Autodesk Inventor part; units mm, degrees
ref_plane "YZ Plane" through (0, 0, 0) normal (1, 0, 0) x (0, 1, 0)
ref_plane "XZ Plane" through (0, 0, 0) normal (0, 1, 0) x (-1, 0, 0)
ref_plane "XY Plane" through (0, 0, 0) normal (0, 0, 1) x (1, 0, 0)
sketch "Sketch1" plane through (0, 0, 0) normal (0, 1, 0) x (-1, 0, 0)
  line L0 (0, 0) -> (127, 0)
  line L1 (127, 0) -> (127, -25.4)
  line L2 (127, -25.4) -> (0, -25.4)
  line L3 (0, -25.4) -> (0, 0)
  dimension "d0" = 127
  dimension "d1" = 25.4
extrude "Extrusion1" add sketch "Sketch1" along normal blind 7.62
sketch "Sketch2" plane through (0, 7.62, 0) normal (0, 1, 0) x (1, 0, 0)
  circle A0 centre (-17.78, 12.7) radius 6.2865
  circle A1 centre (-35.56, 12.7) radius 6.35
  circle A2 centre (-53.34, 12.7) radius 6.4135
  circle A3 centre (-71.12, 12.7) radius 6.477
  circle A4 centre (-88.9, 12.7) radius 6.5405
  circle A5 centre (-106.68, 12.7) radius 6.604
  line L0 (0, 0) -> (0, 25.4)
  dimension "d4" = 12.573
  dimension "d5" = 12.7
  dimension "d6" = 12.827
  dimension "d7" = 12.954
  dimension "d8" = 13.081
  dimension "d9" = 13.208
  dimension "d10" = 17.78
  dimension "d11" = 17.78
  dimension "d12" = 17.78
  dimension "d13" = 17.78
  dimension "d14" = 17.78
  dimension "d15" = 17.78
extrude "Extrusion2" cut sketch "Sketch2" against normal through all
fillet "Fillet1" radius 3.175 4 edges at (-63.5, 7.62, 0) (-63.5, 7.62, -25.4) (0, 7.62, -12.7) (-127, 7.62, -12.7)
properties part number "Bearing hole test"
Geometry check sheet. Reference: the model listing, model coordinates, mm. Give positions to 0.01 mm unless a question says otherwise; leave off trailing zeros. Loops run counter-clockwise (first coordinate to the right, second up) from the corner with the lowest first, then second, coordinate; pieces in that order, holes last. Notation, with made-up numbers: M -14,-2.5 L 2,-2.5 A26 cw 2,27.5 Z; hole C -5.75,25 d1. An arc over 180 degrees is marked long. Answer as CSV lines item,"result".
Item 1: Cross-section at A-A on z = -12.7. Count the separate pieces of the cut face and the enclosed holes in it, and give its area (3 significant figures).
Values:
separate pieces,"7"
enclosed holes,"0"
area,"374 mm²"
Item 2: Cross-section at C-C on y = 2. Record the cut outline in (x, z), and give its area (3 significant figures).
Values:
outline,"M -127,-25.4 L 0,-25.4 L 0,0 L -127,0 Z; hole C -106.68,-12.7 d13.21; hole C -88.9,-12.7 d13.08; hole C -71.12,-12.7 d12.95; hole C -53.34,-12.7 d12.83; hole C -35.56,-12.7 d12.7; hole C -17.78,-12.7 d12.57"
area,"2,440 mm²"
Item 3: Release check for a two-part mould opening along Z. For faces 1 (the cylindrical face through (-95.434, 3.863, -12.988)), 2 (the flat face through (-63, 0, -13)), 3 (the cylindrical face through (-22.41, 3.86, -16.95)), 4 (the cylindrical face through (-62.61, 6.67, -24.49)) record: pulls with the +Z half, pulls with the -Z half, needs draft (parallel to the pull), parting line crosses it, or undercut.
Values:
face 1,"undercut"
face 2,"needs draft"
face 3,"undercut"
face 4,"pulls with the -Z half"
Item 4: Material ranges on line 1 (Z direction, x = -71.12, y = 3); line 2 (Z direction, x = -53.34, y = 5.25); line 3 (Y direction, x = -82.5, z = -3), recorded low to high.
Values:
line 1,"z = -25.4 to -19.18, -6.22 to 0"
line 2,"z = -25.3 to -19.11, -6.29 to -0.1"
line 3,"y = 0 to 7.62"
Item 5: Cross-section at D-D on x = -106.68. Record the cut outline in (y, z) (3 decimals), and give its area (3 significant figures).
Values:
outline,"M 0,-25.4 L 4.445,-25.4 A3.175 ccw 7.62,-22.225 L 7.62,-19.304 L 0,-19.304 Z; M 0,-6.096 L 7.62,-6.096 L 7.62,-3.175 A3.175 ccw 4.445,0 L 0,0 Z"
area,"88.6 mm²"
Item 6: Cross-section at B-B on x = -35.56. Record the cut outline in (y, z) (3 decimals).
Values:
outline,"M 0,-25.4 L 4.445,-25.4 A3.175 ccw 7.62,-22.225 L 7.62,-19.05 L 0,-19.05 Z; M 0,-6.35 L 7.62,-6.35 L 7.62,-3.175 A3.175 ccw 4.445,0 L 0,0 Z"
